```python
from build123d import *

# Parameters (mm, degrees)
SKETCH_1_W          = 223
SKETCH_1_H          = 80
EXTRUDE_1_DEPTH     = 10
SKETCH_3_OUTSIDE_W  = 272.426
SKETCH_3_OUTSIDE_H  = 59.426
CUT_EXTRUDE_1_DEPTH = 138.594512972
CUT_EXTRUDE_2_DEPTH = 119.879140306
CUT_EXTRUDE_3_DEPTH = 119.879140306
SKETCH_7_W          = 14.212670403
SKETCH_7_H          = 6.5
CUT_EXTRUDE_4_DEPTH = 153.966188104
SKETCH_9_W          = 65
SKETCH_9_H          = 6.5
CUT_EXTRUDE_6_DEPTH = 119.799200334
SKETCH_10_W         = 0.633237791
SKETCH_10_H         = 6.5
CUT_EXTRUDE_7_DEPTH = 154.59483235
CUT_EXTRUDE_8_DEPTH = 119.799200334
CUT_EXTRUDE_9_DEPTH = 119.799200334
EXTRUDE_2_DEPTH     = 1


with BuildPart() as part:
    # 스케치1 → 보스-돌출1 (new body)
    with BuildSketch(Plane(origin=(0, 0, 0), x_dir=(1, 0, 0), z_dir=(0, 1, 0))):
        Rectangle(SKETCH_1_W, SKETCH_1_H)
    extrude(amount=EXTRUDE_1_DEPTH)

    # 스케치3 outside → 컷-돌출1 (cut, through all)
    with BuildSketch(Plane.XY.offset(40)):
        with Locations((0, 5)):
            Rectangle(SKETCH_3_OUTSIDE_W, SKETCH_3_OUTSIDE_H)
        Polygon((-111.5, 10), (-111.5, 9), (-84.5, 9), (-73.5, 0), (111.5, 0), (111.5, 1), (-73.5, 1), (-84.5, 10), align=None, mode=Mode.SUBTRACT)
    extrude(amount=-CUT_EXTRUDE_1_DEPTH, mode=Mode.SUBTRACT)

    # 스케치5 → 컷-돌출2 (cut, through all)
    with BuildSketch(Plane(origin=(0, 10, 0), x_dir=(1, 0, 0), z_dir=(0, 1, 0))):
        with BuildLine():
            Line((-111.5, 40), (-111.5, 35.029307783))
            ThreePointArc((-111.5, 35.029307783), (-110.044117957, 38.544117957), (-106.529307783, 40))
            Line((-106.529307783, 40), (-111.5, 40))
        make_face()
        with BuildLine():
            ThreePointArc((-106.529307783, -40), (-110.044117957, -38.544117957), (-111.5, -35.029307783))
            Line((-111.5, -35.029307783), (-111.5, -40))
            Line((-111.5, -40), (-106.529307783, -40))
        make_face()
    extrude(amount=-CUT_EXTRUDE_2_DEPTH, mode=Mode.SUBTRACT)

    # 스케치6 → 컷-돌출3 (cut, through all)
    with BuildSketch(Plane(origin=(0, 10, 0), x_dir=(1, 0, 0), z_dir=(0, 1, 0))):
        Polygon((-106.529307783, 40), (-84.5, 33.5), (-84.5, 40), align=None)
        Polygon((-84.5, -40), (-84.5, -33.5), (-106.529307783, -40), align=None)
    extrude(amount=-CUT_EXTRUDE_3_DEPTH, mode=Mode.SUBTRACT)

    # 스케치7 → 컷-돌출4 (cut, through all)
    with BuildSketch(Plane(origin=(-28.982673267, -35.423267327, 0), x_dir=(0.7739572992033207, -0.6332377902572633, 0), z_dir=(0.6332377902572633, 0.7739572992033207, 0))):
        with Locations((-64.625434484, -36.75)):
            Rectangle(SKETCH_7_W, SKETCH_7_H)
        with Locations((-64.625434484, 36.75)):
            Rectangle(SKETCH_7_W, SKETCH_7_H)
    extrude(amount=-CUT_EXTRUDE_4_DEPTH, mode=Mode.SUBTRACT)

    # 스케치9 → 컷-돌출6 (cut, through all)
    with BuildSketch(Plane(origin=(0, 1, 0), x_dir=(1, 0, 0), z_dir=(0, 1, 0))):
        with Locations((-41, 36.75)):
            Rectangle(SKETCH_9_W, SKETCH_9_H)
        with Locations((-41, -36.75)):
            Rectangle(SKETCH_9_W, SKETCH_9_H)
    extrude(amount=-CUT_EXTRUDE_6_DEPTH, mode=Mode.SUBTRACT)

    # 스케치10 → 컷-돌출7 (cut, through all)
    with BuildSketch(Plane(origin=(-29.472772277, -36.022277228, 0), x_dir=(0.7739572992033206, -0.6332377902572633, 0), z_dir=(-0.6332377902572633, -0.7739572992033206, 0))):
        with Locations((-57.202480386, -36.75)):
            Rectangle(SKETCH_10_W, SKETCH_10_H)
        with Locations((-57.202480386, 36.75)):
            Rectangle(SKETCH_10_W, SKETCH_10_H)
    extrude(amount=-CUT_EXTRUDE_7_DEPTH, mode=Mode.SUBTRACT)

    # 스케치11 → 컷-돌출8 (cut, through all)
    with BuildSketch(Plane(origin=(0, 1, 0), x_dir=(1, 0, 0), z_dir=(0, 1, 0))):
        Polygon((-8.5, -40), (58.5, -40), (-8.5, -33.5), align=None)
        Polygon((-8.5, 33.5), (58.5, 40), (-8.5, 40), align=None)
    extrude(amount=-CUT_EXTRUDE_8_DEPTH, mode=Mode.SUBTRACT)

    # 스케치12 → 컷-돌출9 (cut, through all)
    with BuildSketch(Plane(origin=(0, 1, 0), x_dir=(1, 0, 0), z_dir=(0, 1, 0))):
        with BuildLine():
            Line((111.5, 40), (106.53, 40))
            ThreePointArc((106.53, 40), (110.044320702, 38.544320702), (111.5, 35.03))
            Line((111.5, 35.03), (111.5, 40))
        make_face()
        with BuildLine():
            Line((111.5, -40), (111.5, -35.03))
            ThreePointArc((111.5, -35.03), (110.044320702, -38.544320702), (106.53, -40))
            Line((106.53, -40), (111.5, -40))
        make_face()
    extrude(amount=-CUT_EXTRUDE_9_DEPTH, mode=Mode.SUBTRACT)

    # 스케치13 → 보스-돌출2 (add)
    with BuildSketch(Plane(origin=(0, 1, 0), x_dir=(1, 0, 0), z_dir=(0, 1, 0))):
        with BuildLine():
            Line((-29.5, 33.5), (-63.5, 33.5))
            ThreePointArc((-63.5, 33.5), (-46.5, 16.5), (-29.5, 33.5))
        make_face()
        with BuildLine():
            ThreePointArc((-29.5, 33.5), (-46.5, 50.5), (-63.5, 33.5))
            Line((-63.5, 33.5), (-29.5, 33.5))
        make_face()
        with BuildLine():
            ThreePointArc((-29.5, -33.5), (-46.5, -16.5), (-63.5, -33.5))
            Line((-63.5, -33.5), (-29.5, -33.5))
        make_face()
        with BuildLine():
            Line((-29.5, -33.5), (-63.5, -33.5))
            ThreePointArc((-63.5, -33.5), (-46.5, -50.5), (-29.5, -33.5))
        make_face()
    extrude(amount=-EXTRUDE_2_DEPTH)


solid = part.part
```
For this review, take the finished solid that the model builds, in its own axes (mm). A direction names the side the tool comes from. Round coordinates to 2 decimals unless told otherwise and drop trailing zeros. Write each loop counter-clockwise with the first axis right and the second up, starting at its lowest first coordinate (ties: lowest second). Pieces come first, ordered by that corner, then holes. Notation, with made-up numbers: M 48.5,-38 L 58.5,-38 A34 cw 58.5,1 Z; hole C -18.5,9 d3. An arc over 180 degrees is marked long. One line per item, written item: value. Start each with the question number.
(1) We need section B-B (x = -46.5). Give the boundary of the cut face in (y, z), and give its area (3 significant figures).
(2) We need section C-C (y = 7.25). Give the boundary of the cut face in (x, z), and give its area (3 significant figures).
(3) Machinability: for faces 1 (the flat face through (-98, 10, -1)), 2 (the flat face through (24.5, 0.5, -36.7)), 3 (the flat face through (25.5, 0.5, 36.8)), 4 (the flat face through (18, 1, -1)), 5 (the flat face through (-98, 9, 1)), which of the approach directions +Z, -Z, +X, -X, +Y, -Y give a long, thin tool a straight path to every point of the face, cutting with its end or side? Answer none if there is none.
(4) Wall thickness on line 1 (Y direction, x = -28, z = -29); line 2 (Y direction, x = -97, z = -17); line 3 (X direction, y = 2.25, z = -19): over which ranges is each line inside the solid? List them lowest first.
(5) Insertion check: pin 1 (1.5 mm diameter, centred on x = -36, y = 1.5, fed in from -Z); pin 2 (5 mm diameter, centred on y = 3.5, z = -15.5, fed in from -X); pin 3 (0.5 mm diameter, centred on x = -15, y = 0.5, fed in from -Z); pin 4 (3 mm diameter, centred on x = 88.5, z = 28.5, fed in from -Y). Each pin has a flat end and moves straight along its axis. Give the tip position at first contact, or say it passes through.
(6) We need section A-A (z = 14). Give the boundary of the cut face in (x, y).
Result:
1. outline: M 0,-50.5 L 1,-50.5 L 1,50.5 L 0,50.5 Z
1. area: 101 mm²
2. outline: M -82.36,-33.5 L -81.14,-33.5 L -81.14,33.5 L -82.36,33.5 Z
2. area: 81.9 mm²
3. face 1: +Z, -Z, +X, -X, +Y
3. face 2: -Z, +Y, -Y
3. face 3: +Z, +Y, -Y
3. face 4: +Z, -Z, +X, +Y
3. face 5: +Z, -Z, -X, -Y
4. line 1: 0 to 1
4. line 2: 9 to 10
4. line 3: -76.25 to -75.03
5. pin 1: z = -47.29
5. pin 2: x = -80.83
5. pin 3: z = -33.5
5. pin 4: y = 0
6. outline: M -111.5,9 L -84.5,9 L -73.5,0 L 111.5,0 L 111.5,1 L -73.5,1 L -84.5,10 L -111.5,10 Z
